Build history of the part. All positions in model axes, mm. A direction names the side the tool comes from. Give positions to 0.01 mm unless a question says otherwise; leave off trailing zeros. Order: outer loops, then holes, each group sorted by start corner. A loop starts at its lowest first (then second) coordinate and runs counter-clockwise, first axis right, second up. Notation, with made-up numbers: (35.25, 35) -> (70.25, 35) arc R30 ccw to (70.25, 67) -> close; hole circle Ø10 at (-31.75, 60). An arc over 180 degrees is marked (long way). One line per item, written item: value. Start each with the question number.
(1) Saw through at B-B on z = 0. Give the cut face in (x, y), plus the area to 3 significant figures.
(2) Which spindle directions (+Z, -Z, +X, -X, +Y, -Y) get a long thin tool onto all of the face, cutting with end or side? Do faces 1 (the flat face through (-13, 0, -8)), 2 (the cylindrical face through (-13, 6, 0)). Say none if no direction does.
(3) Saw through at D-D on x = 0. Give the cut face in (y, z), plus the area to 3 significant figures.
(4) Saw through at C-C on y = 7.5. Give the cut face in (x, z).
(5) Probe line 1 (X direction, y = 7.5, z = -0.25); line 2 (X direction, y = 5.5, z = -3.5); line 3 (Z direction, x = -13, y = 3.25). List the from-to ranges inside material, lowest first.
(6) Pin check, flat tips, straight feed: pin 1 (2 mm diameter, centred on x = -2, z = 1, fed in from -Y); pin 2 (1.5 mm diameter, centred on y = 3.5, z = 3, fed in from -X). Stop position of each tip, or through.
(7) Two-plate mould, pull along X, no slides. Class faces 3 (the flat face through (20, 9, 0)), 4 (the cylindrical face through (0.2, 10.5, 0.1)), 5 (the flat face through (2, 11, 9)): +X half, -X half, draft (parallel to the pull), parting line (faces both ways), or undercut.
(8) Saw through at A-A on y = 2.5. Give the cut face in (x, z), plus the area to 3 significant figures.
```python
from build123d import *

# Parameters (mm, degrees)
SKETCH1_W           = 40
SKETCH1_H           = 18
BOSS_EXTRUDE1_DEPTH = 18.47
CUT_EXTRUDE1_REACH  = 20
SKETCH2_R           = 10.5
CUT_EXTRUDE3_REACH  = 42
SKETCH4_R           = 6
CUT_EXTRUDE4_REACH  = 20.47
SKETCH5_W           = 5
SKETCH5_H           = 18


with BuildPart() as part:
    # Sketch1 → Boss-Extrude1 (new body)
    with BuildSketch(Plane(origin=(0, 0, 0), x_dir=(1, 0, 0), z_dir=(0, 1, 0))):
        Rectangle(SKETCH1_W, SKETCH1_H)
    extrude(amount=BOSS_EXTRUDE1_DEPTH)

    # Sketch2 → Cut-Extrude1 (cut, up to next)
    with BuildSketch(Plane.XY.offset(9), mode=Mode.PRIVATE) as cut_extrude1_sk1:
        Circle(SKETCH2_R)
    cut_extrude1_tool1 = extrude(cut_extrude1_sk1.sketch, amount=-CUT_EXTRUDE1_REACH, mode=Mode.PRIVATE) & part.part
    add(cut_extrude1_tool1.solids().sort_by_distance((0, 0, 9))[0], mode=Mode.SUBTRACT)

    # Sketch4 → Cut-Extrude3 (cut, up to next)
    with BuildSketch(Plane.ZY.offset(20), mode=Mode.PRIVATE) as cut_extrude3_sk1:
        Circle(SKETCH4_R)
    cut_extrude3_tool1 = extrude(cut_extrude3_sk1.sketch, amount=-CUT_EXTRUDE3_REACH, mode=Mode.PRIVATE) & part.part
    add(cut_extrude3_tool1.solids().sort_by_distance((-20, 0, 0))[0], mode=Mode.SUBTRACT)

    # Sketch5 → Cut-Extrude4 (cut, up to next)
    with BuildSketch(Plane.XZ, mode=Mode.PRIVATE) as cut_extrude4_sk1:
        with Locations((-17.5, 0)):
            Rectangle(SKETCH5_W, SKETCH5_H)
    cut_extrude4_tool1 = extrude(cut_extrude4_sk1.sketch, amount=-CUT_EXTRUDE4_REACH, mode=Mode.PRIVATE) & part.part
    add(cut_extrude4_tool1.solids().sort_by_distance((-17.5, 0, 0))[0], mode=Mode.SUBTRACT)


solid = part.part
```
Results below:
1. outline: (-15, 6) -> (-8.62, 6) arc R10.5 cw to (10.5, 0) -> (20, 0) -> (20, 18.47) -> (-15, 18.47) -> close
1. area: 443 mm²
2. face 1: +Z, -Z, +X, -X, -Y
2. face 2: -X, -Y
3. outline: (10.5, -9) -> (18.47, -9) -> (18.47, 9) -> (10.5, 9) -> close
3. area: 143 mm²
4. outline: (-15, -9) -> (-7.35, -9) -> (-7.35, 9) -> (-15, 9) -> close; (7.35, -9) -> (20, -9) -> (20, 9) -> (7.35, 9) -> close
5. line 1: x = -15 to -7.35, 7.35 to 20
5. line 2: x = -15 to -8.94, 8.94 to 20
5. line 3: z = -9 to -5.04, 5.04 to 9
6. pin 1: stops at y = 10.06
6. pin 2: stops at x = 9.6
7. face 3: +X half
7. face 4: undercut
7. face 5: draft
8. outline: (-15, -9) -> (-10.2, -9) -> (-10.2, -5.45) -> (-15, -5.45) -> close; (-15, 5.45) -> (-10.2, 5.45) -> (-10.2, 9) -> (-15, 9) -> close; (10.2, -9) -> (20, -9) -> (20, 9) -> (10.2, 9) -> close
8. area: 210 mm²
